```python
from build123d import *

# Parameters (mm, degrees)
SKETCH1_W           = 119
SKETCH1_H           = 114
BOSS_EXTRUDE1_DEPTH = 41
SKETCH4_R           = 4.214519236
CUT_EXTRUDE1_DEPTH  = 41
SKETCH7_R           = 7
CUT_EXTRUDE2_DEPTH  = 35
SKETCH8_R           = 4
CUT_EXTRUDE3_DEPTH  = 55
SKETCH9_R           = 12.7
CUT_EXTRUDE4_DEPTH  = 14
SKETCH10_OUTSIDE_W  = 154.964
SKETCH10_OUTSIDE_H  = 149.964
SKETCH10_OUTSIDE_R  = 50.8
CUT_EXTRUDE5_DEPTH  = 55


with BuildPart() as part:
    # Sketch1 → Boss-Extrude1 (new body)
    with BuildSketch(Plane.XY):
        Rectangle(SKETCH1_W, SKETCH1_H)
    extrude(amount=BOSS_EXTRUDE1_DEPTH)

    # Sketch4 → Cut-Extrude1 (cut)
    with BuildSketch(Plane(origin=(0, 0, 0), x_dir=(-1, 0, 0), z_dir=(0, 0, -1))):
        with Locations((0, 37.6)):
            Circle(SKETCH4_R)
        with Locations((35.759725013, 11.619038988)):
            Circle(SKETCH4_R)
        with Locations((22.100725486, -30.419038988)):
            Circle(SKETCH4_R)
        with Locations((-22.100725486, -30.419038988)):
            Circle(SKETCH4_R)
        with Locations((-35.759725013, 11.619038988)):
            Circle(SKETCH4_R)
    extrude(amount=-CUT_EXTRUDE1_DEPTH, mode=Mode.SUBTRACT)

    # Sketch7 → Cut-Extrude2 (cut)
    with BuildSketch(Plane(origin=(0, 0, 0), x_dir=(-1, 0, 0), z_dir=(0, 0, -1))):
        with Locations((0, 37.6)):
            Circle(SKETCH7_R)
        with Locations((35.759725013, 11.619038988)):
            Circle(SKETCH7_R)
        with Locations((22.100725486, -30.419038988)):
            Circle(SKETCH7_R)
        with Locations((-22.100725486, -30.419038988)):
            Circle(SKETCH7_R)
        with Locations((-35.759725013, 11.619038988)):
            Circle(SKETCH7_R)
    extrude(amount=-CUT_EXTRUDE2_DEPTH, mode=Mode.SUBTRACT)

    # Sketch8 → Cut-Extrude3 (cut)
    with BuildSketch(Plane(origin=(0, 0, 0), x_dir=(-1, 0, 0), z_dir=(0, 0, -1))):
        with Locations((-17.67766953, 17.67766953)):
            Circle(SKETCH8_R)
    extrude(amount=-CUT_EXTRUDE3_DEPTH, mode=Mode.SUBTRACT)

    # Sketch9 → Cut-Extrude4 (cut)
    with BuildSketch(Plane.XY.offset(41)):
        Circle(SKETCH9_R)
    extrude(amount=-CUT_EXTRUDE4_DEPTH, mode=Mode.SUBTRACT)

    # Sketch10 outside → Cut-Extrude5 (cut)
    with BuildSketch(Plane(origin=(0, 0, 0), x_dir=(-1, 0, 0), z_dir=(0, 0, -1))):
        Rectangle(SKETCH10_OUTSIDE_W, SKETCH10_OUTSIDE_H)
        Circle(SKETCH10_OUTSIDE_R, mode=Mode.SUBTRACT)
    extrude(amount=-CUT_EXTRUDE5_DEPTH, mode=Mode.SUBTRACT)


solid = part.part
```
Geometry check sheet. Reference: the model listing, model coordinates, mm. A direction names the side the tool comes from. Round coordinates to 2 decimals unless told otherwise and drop trailing zeros. Loops run counter-clockwise (first coordinate to the right, second up) from the corner with the lowest first, then second, coordinate; pieces in that order, holes last. Notation, with made-up numbers: (24, 70) -> (83, 70) arc R31 cw to (83, 102) -> close; hole circle Ø3 at (86, 58.5). An arc over 180 degrees is marked (long way). Use a Markdown table: item, result.
(1) Sectioned sample at A-A (x = 0). Enter the section's corners in (y, z).
Calculated:
| item | result |
|---|---|
| outline | (-50.8, 0) -> (30.6, 0) -> (30.6, 35) -> (33.39, 35) -> (33.39, 41) -> (12.7, 41) -> (12.7, 27) -> (-12.7, 27) -> (-12.7, 41) -> (-50.8, 41) -> close; (41.81, 35) -> (44.6, 35) -> (44.6, 0) -> (50.8, 0) -> (50.8, 41) -> (41.81, 41) -> close |
(2) Sectioned sample at B-B (y = 0). Enter the section's corners in (x, z).
Calculated:
| item | result |
|---|---|
| outline | (-50.8, 0) -> (50.8, 0) -> (50.8, 41) -> (12.7, 41) -> (12.7, 27) -> (-12.7, 27) -> (-12.7, 41) -> (-50.8, 41) -> close |
(3) Go/stop test with flat-tipped pins: P1, Ø1, axis at y = -20.5, z = 33, coming from the +X side; P2, Ø8, axis at x = -23, z = 10.5, coming from the +Y side; P3, Ø1.5, axis at y = 3, z = 24.5, coming from the +X side; P4, Ø6.5, axis at x = 35.76, y = 11.62, coming from the +Z side. Record where each tip stops, or that it passes through.
Calculated:
| item | result |
|---|---|
| P1 | x = 46.7 |
| P2 | y = 47.11 |
| P3 | x = 50.75 |
| P4 | through |
(4) Sectioned sample at C-C (x = 24). Enter the section's corners in (y, z).
Calculated:
| item | result |
|---|---|
| outline | (-44.77, 0) -> (-37.16, 0) -> (-37.16, 35) -> (-34.18, 35) -> (-34.18, 41) -> (-44.77, 41) -> close; (-26.66, 35) -> (-23.68, 35) -> (-23.68, 0) -> (44.77, 0) -> (44.77, 41) -> (-26.66, 41) -> close |
(5) Sectioned sample at D-D (x = 11). Enter the section's corners in (y, z), then the cut area to 3 significant figures.
Calculated:
| item | result |
|---|---|
| outline | (-49.59, 0) -> (49.59, 0) -> (49.59, 41) -> (6.35, 41) -> (6.35, 27) -> (-6.35, 27) -> (-6.35, 41) -> (-49.59, 41) -> close |
| area | 3,890 mm² |
(6) Scan lines: probe 1 along X at (y, z) = (-36, 21); probe 2 along X at (y, z) = (7, 20.5); probe 3 along Y at (x, z) = (-41.5, 4.5). Record each from-to range of solid material in increasing order.
Calculated:
| item | result |
|---|---|
| probe 1 | -35.84 to -26.33, -17.88 to 17.88, 26.33 to 35.84 |
| probe 2 | -50.32 to -41.02, -30.5 to 30.5, 41.02 to 50.32 |
| probe 3 | -29.3 to 7.61, 15.63 to 29.3 |
(7) Set-up check for faces 1 (the cylindrical face through (-2.75, -12.4, 34.1)), 2 (the cylindrical face through (-3.763, 43.502, 17.255)), 3 (the cylindrical face through (-31.55, 11.8, 37.96)): record each of +Z, -Z, +X, -X, +Y, -Y from which the full face is reachable in a straight line by a thin tool's end or side.
Calculated:
| item | result |
|---|---|
| face 1 | +Z |
| face 2 | -Z |
| face 3 | +Z, -Z |
(8) Mould release check, pull along Y, two halves, no side actions. Record for faces 4 (the cylindrical face through (39.97, 11.8, 37.96)), 5 (the cylindrical face through (11.012, -49.592, 20.213)), 6 (the flat face through (-1, 1, 0)): released by +Y, released by -Y, zero draft, split by the parting line, or undercut.
Calculated:
| item | result |
|---|---|
| face 4 | undercut |
| face 5 | split by the parting line |
| face 6 | zero draft |
